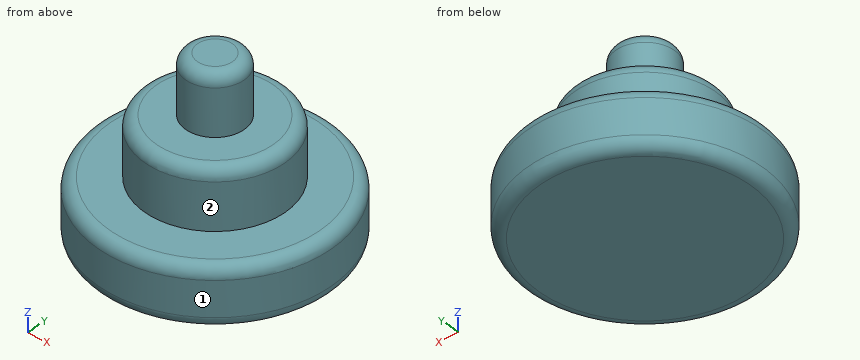
from build123d import *

# Parameters (mm, degrees)
F1_R      = 30
F2_DEPTH  = 25
F0_R      = 50
F2_FACE_R = 30
F3_DEPTH  = 25
F4_R      = 5
F5_R      = 5
F6_R      = 5
F7_R      = 12.5
F8_DEPTH  = 25
F9_R      = 5


with BuildPart() as f2:
    # F1 (on face) → F2 (new body)
    with BuildSketch(Plane.XY):
        Circle(F1_R)
    extrude(amount=F2_DEPTH)

    # F0 (on Top) + F2_face (on face) → F3 (join)
    with BuildSketch(Plane.XY):
        Circle(F0_R)
    with BuildSketch(Plane.XY.offset(25)):
        Circle(F2_FACE_R)
    extrude(amount=F3_DEPTH)

    # F4
    f4_edges = [f2.edges().sort_by_distance(p)[0] for p in [
        (-50, 0, 25),
    ]]
    fillet(f4_edges, radius=F4_R)

    # F5
    f5_edges = [f2.edges().sort_by_distance(p)[0] for p in [
        (-30, 0, 50),
    ]]
    fillet(f5_edges, radius=F5_R)

    # F6
    f6_edges = [f2.edges().sort_by_distance(p)[0] for p in [
        (-50, 0, 0),
    ]]
    fillet(f6_edges, radius=F6_R)

    # F7 (on face) → F8 (join)
    with BuildSketch(Plane.XY.offset(50)):
        Circle(F7_R)
    extrude(amount=F8_DEPTH)

    # F9
    f9_edges = [f2.edges().sort_by_distance(p)[0] for p in [
        (-12.5, 0, 75),
    ]]
    fillet(f9_edges, radius=F9_R)


solid = f2.part
Source: CAD feature listing. Evaluate the final solid. Frame: model axes, mm. Face numbers are marked on the shaded views. A direction names the side the tool comes from. Coordinates: 2 decimals unless noted, no trailing zeros. Loops run counter-clockwise (first coordinate to the right, second up) from the corner with the lowest first, then second, coordinate; pieces in that order, holes last. Notation, with made-up numbers: (-35.5, 40.5) - (14.5, 40.5) arc R24 ccw to (14.5, 79.5) - close; hole circle Ø9 at (73, 3). An arc over 180 degrees is marked (long way). One line per question, with ' | ' between items.
1) Line query: line 1 along Z through (x, y) = (-9, 21); line 2 along Z through (x, y) = (6.5, 42); line 3 along Y through (x, z) = (-2, 61). Output: solid intervals per line, ascending.
Report:
line 1: z = 0 to 50 | line 2: z = 0 to 25 | line 3: y = -12.34 to 12.34
2) Section C-C, the plane z = 55. Return loops of the section in (x, y).
Report:
outline: circle Ø25 at (0, 0)
3) Set-up query: the marked faces 1 and 2. Return all of +Z, -Z, +X, -X, +Y, -Y with unobstructed straight access to the full face (end or side cutting, diameter ignored); none if empty.
Report:
face 1: +Z, -Z | face 2: +Z
4) Section D-D, the plane z = 16. Return loops of the section in (x, y).
Report:
outline: circle Ø100 at (0, 0)
5) Section A-A, the plane y = 0. Return loops of the section in (x, z), then the cut area to 3 significant figures.
Report:
outline: (-50, 5) arc R5 ccw to (-45, 0) - (45, 0) arc R5 ccw to (50, 5) - (50, 20) arc R5 ccw to (45, 25) - (30, 25) - (30, 45) arc R5 ccw to (25, 50) - (12.5, 50) - (12.5, 70) arc R5 ccw to (7.5, 75) - (-7.5, 75) arc R5 ccw to (-12.5, 70) - (-12.5, 50) - (-25, 50) arc R5 ccw to (-30, 45) - (-30, 25) - (-45, 25) arc R5 ccw to (-50, 20) - close | area: 4,580 mm²
6) First-contact query: P1, Ø8, axis at y = -7, z = 28.5, coming from the -X side; P2, Ø5, axis at x = -23, y = 15, coming from the +Z side; P3, Ø6, axis at y = -25, z = 43, coming from the -X side. Flat tips, straight axial feed; report the tip coordinate or a pass-through.
Report:
P1: stops at x = -46.68 | P2: stops at z = 50 | P3: stops at x = -20.4
